Design review of the part built by this model. Coordinates are the model's own, in mm. A direction names the side the tool comes from. Coordinates: 2 decimals unless noted, no trailing zeros. Write each loop counter-clockwise with the first axis right and the second up, starting at its lowest first coordinate (ties: lowest second). Pieces come first, ordered by that corner, then holes. Notation, with made-up numbers: (6, 52) -> (37, 52) arc R34 ccw to (37, 90) -> close; hole circle Ø7 at (16.25, -4.75). An arc over 180 degrees is marked (long way). Answer in a Markdown table with one row per item. Add a question column.
Item 1: For faces 5 (the face through (49.014, 8.851, -9.385)), 6 (the face through (25, -5, -41)), list the 3-axis set-ups (+Z, -Z, +X, -X, +Y, -Y) from which the entire face can be reached by the end or side of a thin tool; tool diameter is ignored.
Item 2: Take a section at A-A, the plane z = -7. Write out the cut boundary in (x, y).
Item 3: Draft analysis for pull direction Z (two halves, no side actions). For faces 1 (the face through (25, 4, 0)), 2 (the face through (25, 5, -80)), 3 (the face through (1, 15, -52)), 4 (the face through (1.014, 8.851, -71.885)), state which applies: released by +Z, released by -Z, zero draft, split by the parting line, or undercut.
Item 4: Take a section at D-D, the plane y = 8.1. Write out the cut boundary in (x, z), and give its area (3 significant figures).
Item 5: Take a section at B-B, the plane y = -3.5. Write out the cut boundary in (x, z), and give its area (3 significant figures).
Item 6: To check wall thickness, follow line 1 (X direction, y = 11.25, z = -7); line 2 (Z direction, x = 4.5, y = 14); line 3 (Y direction, x = 0.65, z = -7). State the ranges of each line that lie inside material, in increasing order.
Item 7: Take a section at C-C, the plane x = 7. Write out the cut boundary in (y, z).
Item 8: Clearance check with flat-ended pins moving along their axes: P1, Ø6, axis at y = 8.1, z = -69.5, coming from the +X side; P2, Ø3, axis at y = 8.1, z = -7, coming from the +X side; P3, Ø2, axis at x = 13.5, z = -52, coming from the +Y side. State where each tip first meets the part, or that it passes through.
from build123d import *

# Parameters (mm, degrees)
SKETCH1_W           = 50
SKETCH1_H           = 80
SKETCH1_W_2         = 46
SKETCH1_H_2         = 76
BOSS_EXTRUDE1_DEPTH = 5
SKETCH1_2_W         = 46
SKETCH1_2_H         = 76
BOSS_EXTRUDE2_DEPTH = 5
SKETCH1_3_W         = 50
SKETCH1_3_H         = 80
SKETCH1_3_W_2       = 46
SKETCH1_3_H_2       = 76
BOSS_EXTRUDE3_DEPTH = 10
SKETCH1_4_W         = 46
SKETCH1_4_H         = 76
CUT_EXTRUDE2_DEPTH  = 49
SKETCH3_R           = 2.5
CUT_EXTRUDE3_DEPTH  = 49
BOSS_EXTRUDE4_START = -5
SKETCH1_5_W         = 46
SKETCH1_5_H         = 76
BOSS_EXTRUDE4_DEPTH = 1
BOSS_EXTRUDE5_START = -5
SKETCH1_6_W         = 50
SKETCH1_6_H         = 80
SKETCH1_6_W_2       = 46
SKETCH1_6_H_2       = 76
BOSS_EXTRUDE5_DEPTH = 1
SKETCH1_7_W         = 50
SKETCH1_7_H         = 80
SKETCH1_7_W_2       = 46
SKETCH1_7_H_2       = 76
BOSS_EXTRUDE6_DEPTH = 15
SKETCH3_2_R         = 2.5
CUT_EXTRUDE4_DEPTH  = 61
FILLET1_R           = 0.5


with BuildPart() as part:
    # Sketch1 → Boss-Extrude1 (new body)
    with BuildSketch(Plane(origin=(0, 0, 0), x_dir=(1, 0, 0), z_dir=(0, 1, 0))):
        with Locations((25, 40)):
            Rectangle(SKETCH1_W, SKETCH1_H)
        with Locations((25, 40)):
            Rectangle(SKETCH1_W_2, SKETCH1_H_2, mode=Mode.SUBTRACT)
    extrude(amount=-BOSS_EXTRUDE1_DEPTH)

    # Sketch1<2> → Boss-Extrude2 (add)
    with BuildSketch(Plane(origin=(0, 0, 0), x_dir=(1, 0, 0), z_dir=(0, 1, 0))):
        with Locations((25, 40)):
            Rectangle(SKETCH1_2_W, SKETCH1_2_H)
    extrude(amount=-BOSS_EXTRUDE2_DEPTH)

    # Sketch1<3> → Boss-Extrude3 (add)
    with BuildSketch(Plane(origin=(0, 0, 0), x_dir=(1, 0, 0), z_dir=(0, 1, 0))):
        with Locations((25, 40)):
            Rectangle(SKETCH1_3_W, SKETCH1_3_H)
        with Locations((25, 40)):
            Rectangle(SKETCH1_3_W_2, SKETCH1_3_H_2, mode=Mode.SUBTRACT)
    extrude(amount=BOSS_EXTRUDE3_DEPTH)

    # Sketch1<4> → Cut-Extrude2 (cut)
    with BuildSketch(Plane(origin=(0, 0, 0), x_dir=(1, 0, 0), z_dir=(0, 1, 0))):
        with Locations((25, 40)):
            Rectangle(SKETCH1_4_W, SKETCH1_4_H)
    extrude(amount=-CUT_EXTRUDE2_DEPTH, mode=Mode.SUBTRACT)

    # Sketch3 → Cut-Extrude3 (cut)
    with BuildSketch(Plane(origin=(50, 0, 0), x_dir=(0, 0, -1), z_dir=(1, 0, 0))):
        with Locations((7, 8.1)):
            Circle(SKETCH3_R)
        with Locations((69.5, 8.1)):
            Circle(SKETCH3_R)
    extrude(amount=-CUT_EXTRUDE3_DEPTH, mode=Mode.SUBTRACT)



with BuildPart() as body_2:
    # Sketch1<5> → Boss-Extrude4 (new body)
    with BuildSketch(Plane(origin=(0, 0, 0), x_dir=(1, 0, 0), z_dir=(0, 1, 0)).offset(BOSS_EXTRUDE4_START)):
        with Locations((25, 40)):
            Rectangle(SKETCH1_5_W, SKETCH1_5_H)
    extrude(amount=-BOSS_EXTRUDE4_DEPTH)


with BuildPart() as part_1:
    add(part.part)

    add(body_2.part)  # Boss-Extrude5 merges body 2
    # Sketch1<6> → Boss-Extrude5 (add)
    with BuildSketch(Plane(origin=(0, 0, 0), x_dir=(1, 0, 0), z_dir=(0, 1, 0)).offset(BOSS_EXTRUDE5_START)):
        with Locations((25, 40)):
            Rectangle(SKETCH1_6_W, SKETCH1_6_H)
        with Locations((25, 40)):
            Rectangle(SKETCH1_6_W_2, SKETCH1_6_H_2, mode=Mode.SUBTRACT)
    extrude(amount=-BOSS_EXTRUDE5_DEPTH)

    # Sketch1<7> → Boss-Extrude6 (add)
    with BuildSketch(Plane(origin=(0, 0, 0), x_dir=(1, 0, 0), z_dir=(0, 1, 0))):
        with Locations((25, 40)):
            Rectangle(SKETCH1_7_W, SKETCH1_7_H)
        with Locations((25, 40)):
            Rectangle(SKETCH1_7_W_2, SKETCH1_7_H_2, mode=Mode.SUBTRACT)
    extrude(amount=BOSS_EXTRUDE6_DEPTH)

    # Sketch3<2> → Cut-Extrude4 (cut)
    with BuildSketch(Plane(origin=(50, 0, 0), x_dir=(0, 0, -1), z_dir=(1, 0, 0))):
        with Locations((7, 8.1)):
            Circle(SKETCH3_2_R)
        with Locations((69.5, 8.1)):
            Circle(SKETCH3_2_R)
    extrude(amount=-CUT_EXTRUDE4_DEPTH, mode=Mode.SUBTRACT)

    # Fillet1
    fillet1_edges = [part_1.edges().sort_by_distance(p)[0] for p in [
        (50, -6, -40),
        (0, -6, -40),
        (25, -6, -80),
        (25, -5, -2),
        (0, 15, -40),
        (25, 15, 0),
        (50, 15, -40),
        (25, 15, -80),
        (0, 4.5, -80),
        (50, 4.5, -80),
        (50, 4.5, 0),
        (0, 4.5, 0),
    ]]
    fillet(fillet1_edges, radius=FILLET1_R)


solid = part_1.part
Answers:
| question | item | result |
|---|---|---|
| 1 | face 5 | +X, -X |
| 1 | face 6 | +Y |
| 2 | outline | (0, -5.5) arc R0.5 ccw to (0.5, -6) -> (49.5, -6) arc R0.5 ccw to (50, -5.5) -> (50, 5.6) -> (48, 5.6) -> (48, -5) -> (2, -5) -> (2, 5.6) -> (0, 5.6) -> close; (0, 10.6) -> (2, 10.6) -> (2, 15) -> (0.5, 15) arc R0.5 ccw to (0, 14.5) -> close; (48, 10.6) -> (50, 10.6) -> (50, 14.5) arc R0.5 ccw to (49.5, 15) -> (48, 15) -> close |
| 3 | face 1 | released by +Z |
| 3 | face 2 | released by -Z |
| 3 | face 3 | zero draft |
| 3 | face 4 | undercut |
| 4 | outline | (0, -79.5) arc R0.5 ccw to (0.5, -80) -> (49.5, -80) arc R0.5 ccw to (50, -79.5) -> (50, -72) -> (48, -72) -> (48, -78) -> (2, -78) -> (2, -72) -> (0, -72) -> close; (0, -67) -> (2, -67) -> (2, -9.5) -> (0, -9.5) -> close; (0, -4.5) -> (2, -4.5) -> (2, -2) -> (48, -2) -> (48, -4.5) -> (50, -4.5) -> (50, -0.5) arc R0.5 ccw to (49.5, 0) -> (0.5, 0) arc R0.5 ccw to (0, -0.5) -> close; (48, -67) -> (50, -67) -> (50, -9.5) -> (48, -9.5) -> close |
| 4 | area | 464 mm^2 |
| 5 | outline | (0, -79.5) arc R0.5 ccw to (0.5, -80) -> (49.5, -80) arc R0.5 ccw to (50, -79.5) -> (50, -0.5) arc R0.5 ccw to (49.5, 0) -> (0.5, 0) arc R0.5 ccw to (0, -0.5) -> close; hole (2, -78) -> (48, -78) -> (48, -2) -> (2, -2) -> close |
| 5 | area | 504 mm^2 |
| 6 | line 1 | x = 0 to 2, 48 to 50 |
| 6 | line 2 | z = -80 to -78, -2 to 0 |
| 6 | line 3 | y = -6 to 5.6, 10.6 to 15 |
| 7 | outline | (-6, -79.5) arc R0.5 ccw to (-5.5, -80) -> (14.5, -80) arc R0.5 ccw to (15, -79.5) -> (15, -78) -> (-5, -78) -> (-5, -2.5) arc R0.5 cw to (-4.5, -2) -> (15, -2) -> (15, -0.5) arc R0.5 ccw to (14.5, 0) -> (-6, 0) -> close |
| 8 | P1 | stops at x = 50 |
| 8 | P2 | passes through |
| 8 | P3 | stops at y = -5 |
